Autodesk Inventor part; units mm, degrees
ref_plane "YZ Plane" through (0, 0, 0) normal (1, 0, 0) x (0, 1, 0)
ref_plane "XZ Plane" through (0, 0, 0) normal (0, 1, 0) x (-1, 0, 0)
ref_plane "XY Plane" through (0, 0, 0) normal (0, 0, 1) x (1, 0, 0)
sketch "Sketch2" plane through (0, 0, 0) normal (0, 0, 1) x (1, 0, 0)
  line L0 (0, 0) -> (42, 0)
  line L1 (42, 0) -> (42, 32)
  line L2 (42, 32) -> (0, 32)
  line L3 (0, 32) -> (0, 0)
  dimension "d0" = 42
  dimension "d1" = 32
extrude "Cover_Body" add sketch "Sketch2" along normal blind 15.8
sketch "Sketch4" plane through (0, 0, 15.8) normal (0, 0, 1) x (1, 0, 0)
  line L0 (42, 32) -> (0, 32)
  line L1 (0, 32) -> (0, 0)
  line L2 (4.5, 24.7) -> (9.5, 24.7)
  line L3 (32.5, 24.7) -> (37.5, 24.7)
  line L4 (42, 0) -> (42, 32)
  line L5 (0, 0) -> (42, 0)
  line L6 (4.5, 24.7) -> (4.5, 27)
  line L7 (4.5, 27) -> (9.5, 27)
  line L8 (9.5, 27) -> (9.5, 32)
  line L9 (37.5, 27) -> (37.5, 24.7)
  line L10 (37.5, 27) -> (32.5, 27)
  line L11 (32.5, 27) -> (32.5, 32)
  line L12 (9.5, 32) -> (32.5, 32)
  line L13 (21, 36.5125) -> (21, -47.625) construction
  line L14 (32.5, 24.7) -> (32.5, 0)
  line L15 (9.5, 24.7) -> (9.5, 0)
  line L16 (9.5, 0) -> (32.5, 0)
  point P0 (4.9935, 32)
  point P1 (37, 32)
  dimension "d6" = 5
  dimension "d14" = 2.3
  dimension "d15" = 2.3
  dimension "d22" = 42
  dimension "d23" = 21
  dimension "d24" = 23
  dimension "d28" = 5
  dimension "d118" = 23
  dimension "d119" = 11.5
  dimension "d120" = 11.5
  dimension "d121" = 24.7
extrude "Servo_Opening" cut sketch "Sketch4" against normal blind 6.3 contours L11 L10 L9 L3 L14 L5 L15 L2 L6 L7 L8 L0
sketch "Sketch5" plane through (0, 0, 15.8) normal (0, 0, 1) x (1, 0, 0)
  line L0 (0, 32) -> (0, 0)
  line L1 (0, 13.2) -> (0, 14.7)
  line L2 (-29.647, 13.95) -> (54.8226, 13.95) construction
  line L3 (0, 0) -> (42, 0)
  line L4 (0, 14.7) -> (9.5, 14.7)
  line L5 (9.5, 14.7) -> (9.5, 13.2)
  line L6 (9.5, 13.2) -> (0, 13.2)
  line L7 (9.5, 0) -> (9.5, 24.7)
  line L8 (9.5, 32) -> (0, 32)
  dimension "d97" = 1.5
  dimension "d131" = 13.2
extrude "Cable_Opening" cut sketch "Sketch5" against normal blind 2.5 contours L4 L5 L6 L0
sketch "Sketch6" plane through (0, 0, 15.8) normal (0, 0, 1) x (1, 0, 0)
  circle A0 centre (3.5, 28) radius 1.25
  circle A1 centre (38.5, 28) radius 1.25
  circle A2 centre (38.5, 4) radius 1.25
  circle A3 centre (3.5, 4) radius 1.25
  line L0 (21, 34.35) -> (21, -13.275) construction
  line L1 (-20.6375, 16) -> (66.675, 16) construction
  line L2 (42, 0) -> (42, 32)
  line L3 (0, 32) -> (0, 0)
  line L4 (9.5, 32) -> (0, 32)
  line L5 (0, 0) -> (42, 0)
  point P0 (42, 12.35)
  point P1 (0, 12.35)
  dimension "d29" = 2.5
  dimension "d30" = 2.5
  dimension "d31" = 2.5
  dimension "d32" = 2.5
  dimension "d33" = 42
  dimension "d34" = 21
  dimension "d35" = 32
  dimension "d36" = 16
  dimension "d37" = 35
  dimension "d38" = 17.5
  dimension "d39" = 24
  dimension "d40" = 12
extrude "Cover_Mounting_Holes" cut sketch "Sketch6" against normal up to surface (15.8 mm away)
sketch "Sketch16" plane through (0, 0, 0) normal (0, 0, -1) x (-1, 0, 0)
  circle A0 centre (-3.5, 4) radius 2.25
  circle A1 centre (-3.5, 4) radius 1.25
  circle A2 centre (-38.5, 4) radius 2.25
  circle A3 centre (-3.5, 28) radius 2.25
  circle A4 centre (-38.5, 28) radius 2.25
  circle A5 centre (-38.5, 4) radius 1.25
  circle A6 centre (-38.5, 28) radius 1.25
  circle A7 centre (-3.5, 28) radius 1.25
  point P0 (0, 0)
  dimension "d98" = 4.5
  dimension "d99" = 4.5
  dimension "d100" = 4.5
  dimension "d101" = 4.5
extrude "Slot_Mounting_ScrewsHead" cut sketch "Sketch16" against normal blind 9
sketch "Sketch17" plane through (0, 0, 9.5) normal (0, 0, 1) x (1, 0, 0)
  circle A0 centre (14.75, 26.6) radius 1.75
  line L0 (9.5, 32) -> (32.5, 32)
  line L1 (9.5, 27) -> (9.5, 32)
  point P0 (0, 0)
  dimension "d105" = 3.5
  dimension "d106" = 5.4
  dimension "d107" = 5.25
extrude "Heat_Dissipation_Hole" cut sketch "Sketch17" against normal up to surface (9.5 mm away)
pattern_linear "Pattern_Heat_Dissipation_Hole" count 3 spacing 6.25 along (1, 0, 0) count 3 spacing 6.25 along (0, -1, 0) of "Heat_Dissipation_Hole"
sketch "Sketch20" plane through (0, 0, 0) normal (0, 0, -1) x (-1, 0, 0)
  line L0 (-42, 0) -> (-42, 32)
  line L1 (0, 0) -> (-42, 0)
  line L2 (-42, 0) -> (-42, 32)
  line L3 (-42, 32) -> (0, 32)
  line L4 (0, 32) -> (0, 0)
extrude "Material reduction for PLA printing only" cut sketch "Sketch20" against normal blind 1
equation "\"d15\" = d14"
equation "\"d23\" = 0.5 * d22"
equation "\"d28\" = d6"
equation "\"d120\" = 0.5 * d118"
equation "\"d34\" = 0.5 * d33"
equation "\"d36\" = 0.5 * d35"
equation "\"d38\" = 0.5 * d37"
equation "\"d40\" = 0.5 * d39"
equation "\"d98\" = d99"
equation "\"d99\" = d101"
equation "\"d100\" = d101"
properties part number "Module_Cover"
The model under review builds one solid part; all positions refer to its coordinate system, in mm. A direction names the side the tool comes from. Give positions to 0.01 mm unless a question says otherwise; leave off trailing zeros. Write each loop counter-clockwise with the first axis right and the second up, starting at its lowest first coordinate (ties: lowest second). Pieces come first, ordered by that corner, then holes.
(1) Tool access review of faces 4 (the flat face through (5, 14.7, 15)), 5 (the flat face through (9.5, 29, 13)), 6 (the cylindrical face through (15.56, 18.8, 5.31)), 7 (the cylindrical face through (1.354, 4.676, 4.944)), 8 (the flat face through (7, 24.7, 13)): name each direction out of +Z, -Z, +X, -X, +Y, -Y from which nothing blocks a thin tool from reaching the whole face with its end or side.
(2) To check wall thickness, follow L1, parallel to Y at x = 14.75, z = 7.5; L2, parallel to X at y = 14, z = 8; L3, parallel to X at y = 2, z = 12. State the ranges of each line that lie inside material, in increasing order.
(3) Consider section B-B, the plane z = 12.25. Give the boundary of the cut face in (x, y), and give its area (3 significant figures).
(4) For P1, Ø3, axis at x = 21, y = 20.35, coming from the -Z side; P2, Ø4, axis at x = 38.5, y = 28, coming from the -Z side; P3, Ø5.5, axis at x = 14.75, y = 20.35, coming from the +Z side, all flat-tipped, find the tip position at first contact; note any pin that passes through.
(5) Consider section D-D, the plane y = 4. Give the boundary of the cut face in (x, z), and give its area (3 significant figures).
(6) The part is to be moulded in two halves that separate along Y. For faces 1 (the flat face through (5, 14, 13.3)), 2 (the flat face through (37, 16, 15.8)), 3 (the flat face through (21, 0, 7)), say which applies: released by +Y, released by -Y, zero draft, split by the parting line, or undercut.
(7) Consider section A-A, the plane y = 14.1. Give the boundary of the cut face in (x, z).
(8) Consider section C-C, the plane x = 27.25. Give the boundary of the cut face in (y, z).
Returned:
1. face 4: +Z, -X
1. face 5: +Z, +Y, -Y
1. face 6: +Z, -Z
1. face 7: -Z
1. face 8: +Z
2. L1: y = 0 to 12.35, 15.85 to 18.6, 22.1 to 24.85, 28.35 to 32
2. L2: x = 0 to 13, 16.5 to 19.25, 22.75 to 25.5, 29 to 42
2. L3: x = 0 to 9.5, 32.5 to 42
3. outline: (0, 0) - (9.5, 0) - (9.5, 24.7) - (4.5, 24.7) - (4.5, 27) - (9.5, 27) - (9.5, 32) - (0, 32) - close; (32.5, 0) - (42, 0) - (42, 32) - (32.5, 32) - (32.5, 27) - (37.5, 27) - (37.5, 24.7) - (32.5, 24.7) - close; hole circle Ø2.5 at (3.5, 4); hole circle Ø2.5 at (3.5, 28); hole circle Ø2.5 at (38.5, 4); hole circle Ø2.5 at (38.5, 28)
3. area: 565 mm2
4. P1: passes through
4. P2: stops at z = 9
4. P3: stops at z = 9.5
5. outline: (0, 1) - (1.25, 1) - (1.25, 9) - (2.25, 9) - (2.25, 15.8) - (0, 15.8) - close; (4.75, 9) - (5.75, 9) - (5.75, 1) - (36.25, 1) - (36.25, 9) - (37.25, 9) - (37.25, 15.8) - (32.5, 15.8) - (32.5, 9.5) - (9.5, 9.5) - (9.5, 15.8) - (4.75, 15.8) - close; (39.75, 9) - (40.75, 9) - (40.75, 1) - (42, 1) - (42, 15.8) - (39.75, 15.8) - close
5. area: 371 mm2
6. face 1: undercut
6. face 2: zero draft
6. face 3: released by -Y
7. outline: (0, 1) - (13, 1) - (13, 9.5) - (9.5, 9.5) - (9.5, 13.3) - (0, 13.3) - close; (16.5, 1) - (19.25, 1) - (19.25, 9.5) - (16.5, 9.5) - close; (22.75, 1) - (25.5, 1) - (25.5, 9.5) - (22.75, 9.5) - close; (29, 1) - (42, 1) - (42, 15.8) - (32.5, 15.8) - (32.5, 9.5) - (29, 9.5) - close
8. outline: (0, 1) - (12.35, 1) - (12.35, 9.5) - (0, 9.5) - close; (15.85, 1) - (18.6, 1) - (18.6, 9.5) - (15.85, 9.5) - close; (22.1, 1) - (24.85, 1) - (24.85, 9.5) - (22.1, 9.5) - close; (28.35, 1) - (32, 1) - (32, 9.5) - (28.35, 9.5) - close
